from build123d import *

# Parameters (mm, degrees)
SKETCH1_W             = 20
SKETCH1_H             = 4
BOSS_EXTRUDE1_DEPTH   = 6
BOSS_EXTRUDE1_2_DEPTH = 6
BOSS_EXTRUDE2_DEPTH   = 6
LPATTERN1_COUNT       = 5
LPATTERN1_PITCH       = 2
SKETCH4_W             = 20
SKETCH4_H             = 10.4
BOSS_EXTRUDE3_DEPTH   = 2
BOSS_EXTRUDE4_DEPTH   = 5


with BuildPart() as part:
    # Sketch1 → Boss-Extrude1 (new body)
    with BuildSketch(Plane(origin=(0, 0, 0), x_dir=(1, 0, 0), z_dir=(0, 1, 0))):
        with Locations((10, 3.2)):
            Rectangle(SKETCH1_W, SKETCH1_H)
    extrude(amount=BOSS_EXTRUDE1_DEPTH)



with BuildPart() as body_2:
    # Sketch1 → Boss-Extrude1 2 (new body)
    with BuildSketch(Plane(origin=(0, 0, 0), x_dir=(1, 0, 0), z_dir=(0, 1, 0))):
        with Locations((10, -3.2)):
            Rectangle(SKETCH1_W, SKETCH1_H)
    extrude(amount=BOSS_EXTRUDE1_2_DEPTH)

    # Sketch3 → Boss-Extrude2 (add)
    with BuildSketch(Plane.XZ):
        with BuildLine():
            Line((17.48035085, -0.4), (18, -0.4))
            ThreePointArc((18, -0.4), (18.098907071, -0.362771412), (18.148718534, -0.269565217))
            ThreePointArc((18.148718534, -0.269565217), (18.182563711, -0.111937846), (18.241299021, 0.038202247))
            ThreePointArc((18.241299021, 0.038202247), (18.740175425, 0.35), (19.23905183, 0.038202247))
            ThreePointArc((19.23905183, 0.038202247), (19.297787139, -0.111937846), (19.331632316, -0.269565217))
            ThreePointArc((19.331632316, -0.269565217), (19.381443779, -0.362771412), (19.48035085, -0.4))
            Line((19.48035085, -0.4), (20, -0.4))
            Line((20, -0.4), (20, 1.2))
            Line((20, 1.2), (17.48035085, 1.2))
            Line((17.48035085, 1.2), (17.48035085, -0.4))
        make_face()
    boss_extrude2 = extrude(amount=-BOSS_EXTRUDE2_DEPTH)

    # LPattern1: Boss-Extrude2 ×5
    with Locations(*[(-i * LPATTERN1_PITCH, 0, 0) for i in range(1, LPATTERN1_COUNT)]):
        add(boss_extrude2)


with BuildPart() as part_1:
    add(part.part)

    add(body_2.part)  # Boss-Extrude3 merges body 2
    # Sketch4 → Boss-Extrude3 (add)
    with BuildSketch(Plane(origin=(0, 6, 0), x_dir=(1, 0, 0), z_dir=(0, 1, 0))):
        with Locations((10, 0)):
            Rectangle(SKETCH4_W, SKETCH4_H)
    extrude(amount=BOSS_EXTRUDE3_DEPTH)

    # Sketch5 → Boss-Extrude4 (add)
    with BuildSketch(Plane(origin=(20, 0, 0), x_dir=(0, 0, -1), z_dir=(1, 0, 0))):
        Polygon((-9.038202247, 26), (8.961797753, 26), (8.961797753, 8), (5.2, 4.08688479), (5.2, 8), (-5.2, 8), (-5.2, 4.161797753), (-9.038202247, 8), align=None)
    extrude(amount=-BOSS_EXTRUDE4_DEPTH)


solid = part_1.part
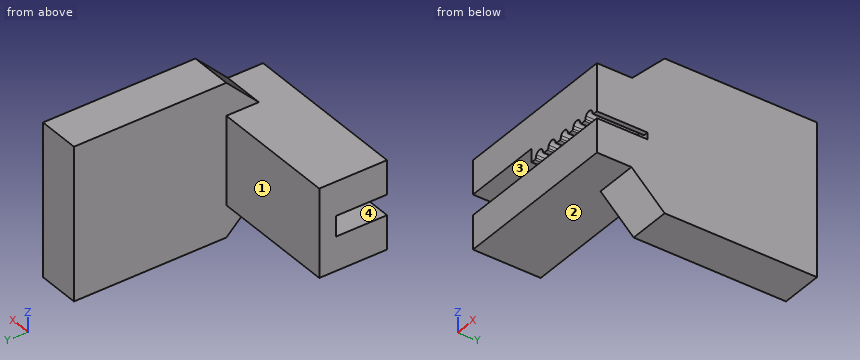
Build history of the part. All positions in model axes, mm. Face numbers are marked on the shaded views. A direction names the side the tool comes from. Give positions to 0.01 mm unless a question says otherwise; leave off trailing zeros. Write each loop counter-clockwise with the first axis right and the second up, starting at its lowest first coordinate (ties: lowest second). Pieces come first, ordered by that corner, then holes. Notation, with made-up numbers: (4.5, 61) - (59.5, 61) arc R10 ccw to (59.5, 72) - close; hole circle Ø8 at (-2, -29.75). An arc over 180 degrees is marked (long way). Use one line per item in the form item = value. Start each with the question number.
1. Band-saw the part on A-A on x = 7.5. Write the cut outline in (y, z), plus the area to 3 significant figures.
2. Band-saw the part on D-D on z = 6.75. Write the cut outline in (x, y).
3. Probe line 1 (Y direction, x = 13, z = -5); line 2 (Z direction, x = 11.5, y = 5.5); line 3 (X direction, y = 14.75, z = 4.5). List the from-to ranges inside material, lowest first. Write a range as [from, to].
4. Drop flat-ended pins along their axis: pin 1 Ø2.5 at (x, y) = (10.5, 2) entering from +Z; pin 2 Ø0.5 at (y, z) = (2, 0) entering from -X; pin 3 Ø0.6 at (x, y) = (13.5, 2) entering from -Z. Give the stop position or say it passes through.
5. 3-axis set-ups, long thin cutter, end or side, ignore diameter. For the marked faces 1, 2, 3 and 4: which of +Z, -Z, +X, -X, +Y, -Y reach the whole face in a straight line?
6. Band-saw the part on C-C on z = -2.75. Write the cut outline in (x, y), plus the area to 3 significant figures.
7. Band-saw the part on B-B on y = 13.75. Write the cut outline in (x, z), plus the area to 3 significant figures.
Conclusion:
q1.outline = (0, -5.2) - (8, -5.2) - (8, 5.2) - (0, 5.2) - (0, 1.2) - (6, 1.2) - (6, -1.2) - (0, -1.2) - close
q1.area = 68.8 mm²
q2.outline = (15, 5.71) - (20, 5.71) - (20, 26) - (15, 26) - close
q3.line_1 = [0, 8]
q3.line_2 = [-5.2, -1.2], [-0.4, 5.2]
q3.line_3 = [15, 20]
q4.pin_1 = 5.2
q4.pin_2 = 9.48
q4.pin_3 = -5.2
q5.face_1 = +Z, -Z, -X, +Y
q5.face_2 = -Z, -X, -Y
q5.face_3 = -X, -Y
q5.face_4 = +X, -X, -Y
q6.outline = (0, 0) - (20, 0) - (20, 26) - (15, 26) - (15, 8) - (0, 8) - close
q6.area = 250 mm²
q7.outline = (15, -8.96) - (20, -8.96) - (20, 9.04) - (15, 9.04) - close
q7.area = 90.0 mm²
